from build123d import *

# Parameters (mm, degrees)
CROQUIS1_R              = 20
SALIENTE_EXTRUIR1_DEPTH = 1
SALIENTE_EXTRUIR2_DEPTH = 1
CORTAR_EXTRUIR1_REACH   = 35.956
CROQUIS4_R              = 1.5


with BuildPart() as part:
    # Croquis1 → Saliente-Extruir1 (new body)
    with BuildSketch(Plane(origin=(0, 0, 0), x_dir=(0, 1, 0), z_dir=(0, 0, 1))):
        with Locations(Location((0, 0, 0), (0, 0, 270))):
            Circle(CROQUIS1_R)
    extrude(amount=SALIENTE_EXTRUIR1_DEPTH)

    # Croquis2 → Saliente-Extruir2 (add)
    with BuildSketch(Plane(origin=(0, 0, 0), x_dir=(0, 1, 0), z_dir=(0, 0, 1))):
        with BuildLine():
            Line((0, -24), (1.47572399, -19.945481661))
            ThreePointArc((1.47572399, -19.945481661), (0, -20), (-1.47572399, -19.945481661))
            Line((-1.47572399, -19.945481661), (0, -24))
        make_face()
        with BuildLine():
            Line((-12, -20.784609691), (-8.694726367, -18.011155804))
            ThreePointArc((-8.694726367, -18.011155804), (-10, -17.320508076), (-11.250755295, -16.535431815))
            Line((-11.250755295, -16.535431815), (-12, -20.784609691))
        make_face()
        with BuildLine():
            Line((-20.784609691, -12), (-16.535431815, -11.250755295))
            ThreePointArc((-16.535431815, -11.250755295), (-17.320508076, -10), (-18.011155804, -8.694726367))
            Line((-18.011155804, -8.694726367), (-20.784609691, -12))
        make_face()
        with BuildLine():
            Line((-24, 0), (-19.945481661, -1.47572399))
            ThreePointArc((-19.945481661, -1.47572399), (-20, 0), (-19.945481661, 1.47572399))
            Line((-19.945481661, 1.47572399), (-24, 0))
        make_face()
        with BuildLine():
            Line((-20.784609691, 12), (-18.011155804, 8.694726367))
            ThreePointArc((-18.011155804, 8.694726367), (-17.320508076, 10), (-16.535431815, 11.250755295))
            Line((-16.535431815, 11.250755295), (-20.784609691, 12))
        make_face()
        with BuildLine():
            Line((-12, 20.784609691), (-11.250755295, 16.535431815))
            ThreePointArc((-11.250755295, 16.535431815), (-10, 17.320508076), (-8.694726367, 18.011155804))
            Line((-8.694726367, 18.011155804), (-12, 20.784609691))
        make_face()
        with BuildLine():
            Line((0, 24), (-1.47572399, 19.945481661))
            ThreePointArc((-1.47572399, 19.945481661), (0, 20), (1.47572399, 19.945481661))
            Line((1.47572399, 19.945481661), (0, 24))
        make_face()
        with BuildLine():
            Line((12, 20.784609691), (8.694726367, 18.011155804))
            ThreePointArc((8.694726367, 18.011155804), (10, 17.320508076), (11.250755295, 16.535431815))
            Line((11.250755295, 16.535431815), (12, 20.784609691))
        make_face()
        with BuildLine():
            Line((20.784609691, 12), (16.535431815, 11.250755295))
            ThreePointArc((16.535431815, 11.250755295), (17.320508076, 10), (18.011155804, 8.694726367))
            Line((18.011155804, 8.694726367), (20.784609691, 12))
        make_face()
        with BuildLine():
            Line((24, 0), (19.945481661, 1.47572399))
            ThreePointArc((19.945481661, 1.47572399), (20, 0), (19.945481661, -1.47572399))
            Line((19.945481661, -1.47572399), (24, 0))
        make_face()
        with BuildLine():
            Line((20.784609691, -12), (18.011155804, -8.694726367))
            ThreePointArc((18.011155804, -8.694726367), (17.320508076, -10), (16.535431815, -11.250755295))
            Line((16.535431815, -11.250755295), (20.784609691, -12))
        make_face()
        with BuildLine():
            Line((12, -20.784609691), (11.250755295, -16.535431815))
            ThreePointArc((11.250755295, -16.535431815), (10, -17.320508076), (8.694726367, -18.011155804))
            Line((8.694726367, -18.011155804), (12, -20.784609691))
        make_face()
    extrude(amount=SALIENTE_EXTRUIR2_DEPTH)

    # Croquis4 → Cortar-Extruir1 (cut, up to next)
    with BuildSketch(Plane.XY.offset(1), mode=Mode.PRIVATE) as cortar_extruir1_sk1:
        with Locations((6, 0)):
            Circle(CROQUIS4_R)
    cortar_extruir1_tool1 = extrude(cortar_extruir1_sk1.sketch, amount=-CORTAR_EXTRUIR1_REACH, mode=Mode.PRIVATE) & part.part
    # Croquis4 → Cortar-Extruir1 (cut, up to next)
    with BuildSketch(Plane.XY.offset(1), mode=Mode.PRIVATE) as cortar_extruir1_sk2:
        with Locations((-6, 0)):
            Circle(CROQUIS4_R)
    cortar_extruir1_tool2 = extrude(cortar_extruir1_sk2.sketch, amount=-CORTAR_EXTRUIR1_REACH, mode=Mode.PRIVATE) & part.part
    add(cortar_extruir1_tool1.solids().sort_by_distance((6, 0, 1))[0], mode=Mode.SUBTRACT)
    add(cortar_extruir1_tool2.solids().sort_by_distance((-6, 0, 1))[0], mode=Mode.SUBTRACT)


solid = part.part
The model under review builds one solid part; all positions refer to its coordinate system, in mm. A direction names the side the tool comes from. Round coordinates to 2 decimals unless told otherwise and drop trailing zeros. Order: outer loops, then holes, each group sorted by start corner. A loop starts at its lowest first (then second) coordinate and runs counter-clockwise, first axis right, second up. Notation, with made-up numbers: (79.25, -32.5) - (85.25, -32.5) arc R14 cw to (85.25, -16.5) - close; hole circle Ø10 at (82, -1). An arc over 180 degrees is marked (long way). Use one line per item in the form item = value.
Q1. Add section C-C on y = -3. Give the boundary of the cut face in (x, z).
Response values:
outline = (-19.77, 0) - (19.77, 0) - (19.77, 1) - (-19.77, 1) - close
Q2. To check wall thickness, follow line 1 (X direction, y = -14.5, z = 0.3); line 2 (Y direction, x = -4, z = 0.3); line 3 (Y direction, x = 6, z = 0.6). State the ranges of each line that lie inside material, in increasing order.
Response values:
line_1 = -13.77 to 13.77
line_2 = -19.6 to 19.6
line_3 = -19.08 to -1.5, 1.5 to 19.08
Q3. Add section B-B on z = 0.15. Give the number of separate pieces and of enclosed holes in the cut face, then the cut area to 3 significant figures.
Response values:
separate_pieces = 1
enclosed_holes = 2
area = 1,310 mm^2
Q4. Add section D-D on y = 21.5. Give the boundary of the cut face in (x, z).
Response values:
outline = (-0.91, 0) - (0.91, 0) - (0.91, 1) - (-0.91, 1) - close
Q5. Mouldability with a two-part tool opening along Y and no side actions: class faces 1 (the flat face through (21.94, -0.75, 0.49)), 2 (the cylindrical face through (5.227, 19.305, 0.493)), 3 (the cylindrical face through (5.13, -19.33, 0.49)) as pulls with the +Y half, pulls with the -Y half, needs draft (parallel to the pull), parting line crosses it, or undercut.
Response values:
face_1 = undercut
face_2 = pulls with the +Y half
face_3 = pulls with the -Y half
Q6. Tool access review of faces 4 (the cylindrical face through (-19.305, 5.227, 0.493)), 5 (the flat face through (-10.324, 19.378, 0.493)), 6 (the flat face through (0, 0, 0)), 7 (the cylindrical face through (19.33, 5.13, 0.49)), 8 (the flat face through (-0.75, -21.94, 0.49)): name each direction out of +Z, -Z, +X, -X, +Y, -Y from which nothing blocks a thin tool from reaching the whole face with its end or side.
Response values:
face_4 = +Z, -Z, -X
face_5 = +Z, -Z, +Y
face_6 = -Z, +X, -X, +Y, -Y
face_7 = +Z, -Z, +X
face_8 = +Z, -Z, -Y
Q7. Add section A-A on x = 6. Give the boundary of the cut face in (y, z), then the cut area to 3 significant figures.
Response values:
outline = (-19.08, 0) - (-1.5, 0) - (-1.5, 1) - (-19.08, 1) - close; (1.5, 0) - (19.08, 0) - (19.08, 1) - (1.5, 1) - close
area = 35.2 mm^2
